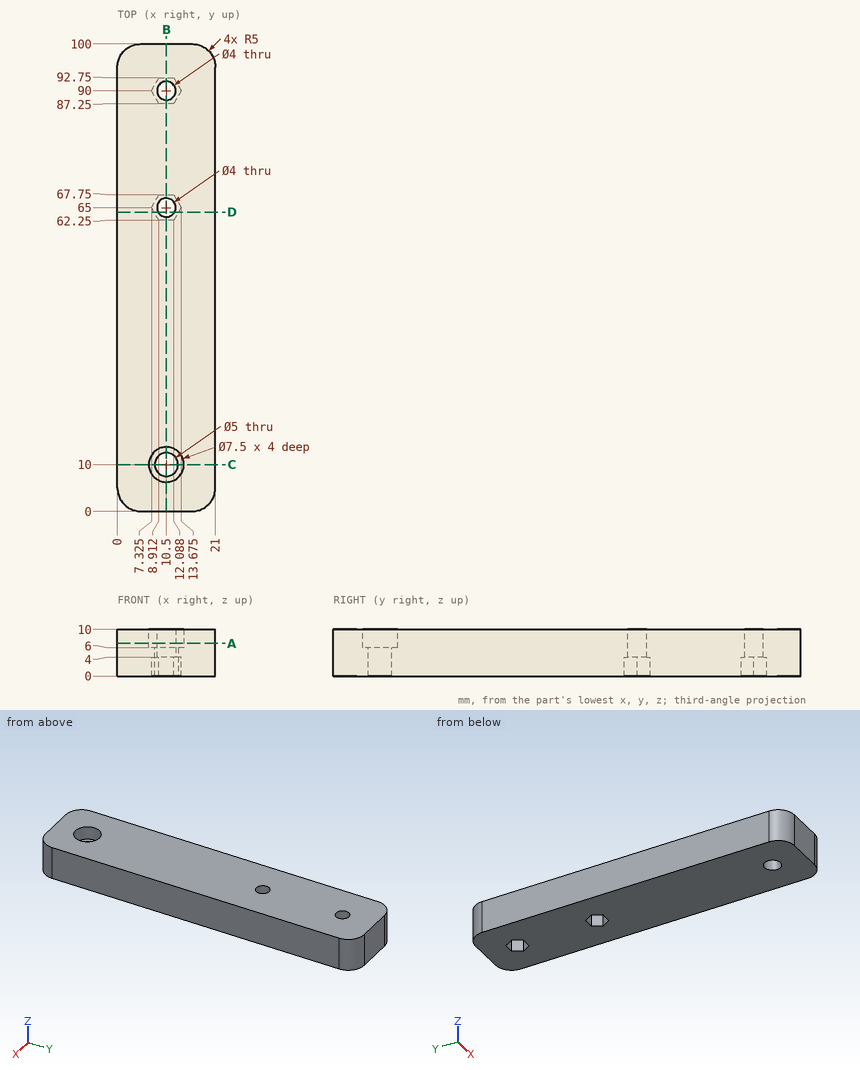
Verification items for this drawing (mm, ordinates from the low corner). Round coordinates to 2 decimals unless told otherwise and drop trailing zeros. Order: outer loops, then holes, each group sorted by start corner. A loop starts at its lowest first (then second) coordinate and runs counter-clockwise, first axis right, second up. Notation, with made-up numbers: (18.25, 59) - (44.25, 59) arc R10 ccw to (44.25, 65) - close; hole circle Ø9 at (73, -6). An arc over 180 degrees is marked (long way). Use CSV: the item, a comma, the result in double quotes. Start each with the question number.
1) Go/stop test with flat-tipped pins: P1, Ø6.5, axis at x = 10.5, y = 10, coming from the -Z side; P2, Ø1.6, axis at x = 10, y = 90, coming from the -Z side. Record where each tip stops, or that it passes through.
2) Section check D-D, the plane y = 64. Record the cut outline in (x, z).
3) Section check B-B, the plane x = 10.5. Record the cut outline in (y, z).
4) Section check C-C, the plane y = 10. Record the cut outline in (x, z), plus the area to 3 significant figures.
5) Section check A-A, the plane z = 7. Record the cut outline in (x, y), plus the area to 3 significant figures.
6) Thickness scan on L1, parallel to Y at x = 10.5, z = 8.3; L2, parallel to Y at x = 10.5, z = 5.4; L3, parallel to X at y = 9, z = 7.75 (1 decimal). Record the ranges inside material, lowest first.
Answers:
1,P1,"stops at z = 0"
1,P2,"passes through"
2,outline,"(0, 0) - (7.9, 0) - (7.9, 4) - (8.77, 4) - (8.77, 10) - (0, 10) - close; (12.23, 4) - (13.1, 4) - (13.1, 0) - (21, 0) - (21, 10) - (12.23, 10) - close"
3,outline,"(0, 0) - (7.5, 0) - (7.5, 6) - (6.25, 6) - (6.25, 10) - (0, 10) - close; (12.5, 0) - (62.25, 0) - (62.25, 4) - (63, 4) - (63, 10) - (13.75, 10) - (13.75, 6) - (12.5, 6) - close; (67, 4) - (67.75, 4) - (67.75, 0) - (87.25, 0) - (87.25, 4) - (88, 4) - (88, 10) - (67, 10) - close; (92, 4) - (92.75, 4) - (92.75, 0) - (100, 0) - (100, 10) - (92, 10) - close"
4,outline,"(0, 0) - (8, 0) - (8, 6) - (6.75, 6) - (6.75, 10) - (0, 10) - close; (13, 0) - (21, 0) - (21, 10) - (14.25, 10) - (14.25, 6) - (13, 6) - close"
4,area,"150 mm²"
5,outline,"(0, 5) arc R5 ccw to (5, 0) - (16, 0) arc R5 ccw to (21, 5) - (21, 95) arc R5 ccw to (16, 100) - (5, 100) arc R5 ccw to (0, 95) - close; hole circle Ø7.5 at (10.5, 10); hole circle Ø4 at (10.5, 65); hole circle Ø4 at (10.5, 90)"
5,area,"2,010 mm²"
6,L1,"y = 0 to 6.25, 13.75 to 63, 67 to 88, 92 to 100"
6,L2,"y = 0 to 7.5, 12.5 to 63, 67 to 88, 92 to 100"
6,L3,"x = 0 to 6.9, 14.1 to 21"
